The listing builds one solid part. Answer for the finished solid, in the listing's coordinates (mm). A direction names the side the tool comes from. Coordinates: 2 decimals unless noted, no trailing zeros. Loops run counter-clockwise (first coordinate to the right, second up) from the corner with the lowest first, then second, coordinate; pieces in that order, holes last. Notation, with made-up numbers: M 38.5,23 L 97.5,23 A12 ccw 97.5,29 Z; hole C 25,69 d4. An arc over 180 degrees is marked long. Answer as a JSON object with one key per item and string values. Group by question number.
1. A cutting plane is placed at A-A on z = 15.5. Give the vertices of the cut face in (x, y), and give its area (3 significant figures).
2. A cutting plane is placed at C-C on x = -2.1. Give the vertices of the cut face in (y, z).
3. A cutting plane is placed at D-D on y = 2.5. Give the vertices of the cut face in (x, z).
4. Straight lines are drawn through the part: L1, parallel to Z at x = -0.6, y = 1.5; L2, parallel to Y at x = 0.7, z = 6.75; L3, parallel to Z at x = 0.1, y = 0.25. For each, find the intervals that lie inside material, in ascending order.
5. A cutting plane is placed at B-B on y = 0. Give the vertices of the cut face in (x, z), and give its area (3 significant figures).
6. Determine the mould class of faces 1 (the face through (0, 2, 6)), 2 (the face through (-1.5, 0.07, 3.08)), 3 (the face through (-0.27, -1.22, 13.4)), 4 (the face through (1.405, -2.48, 13.395)) for opening direction Y: released by +Y, released by -Y, zero draft, split by the parting line, or undercut.
7. For faces 5 (the face through (2.85, 0, 13)), 6 (the face through (0, 0, 6)), determine the directions among +Z, -Z, +X, -X, +Y, -Y from which every point of the face is accessible in a straight line to the end or side of a thin tool.
from build123d import *

# Parameters (mm, degrees)
SKETCH_R     = 1.5
PAD_DEPTH    = 6
SKETCH001_R  = 1.25
PAD001_DEPTH = 15
CHAMFER_SIZE = 0.25


with BuildPart() as part:
    # Sketch → Pad (new body)
    with BuildSketch(Plane.XY):
        Circle(SKETCH_R)
    extrude(amount=PAD_DEPTH)

    # Sketch001 (on Face3 of Pad) → Pad001 (join)
    with BuildSketch(Plane.XY.offset(6)):
        Polygon((0, -3.290897), (2.85, -1.645448), (2.85, 1.645448), (0, 3.290897), (-2.85, 1.645448), (-2.85, -1.645448), align=None)
        Circle(SKETCH001_R, mode=Mode.SUBTRACT)
    extrude(amount=PAD001_DEPTH)

    # Chamfer
    chamfer_edges = [part.edges().sort_by_distance(p)[0] for p in [
        (-1.5, 0, 0),
    ]]
    chamfer(chamfer_edges, length=CHAMFER_SIZE)


solid = part.part
From the geometry:
{
 "1": {"outline": "M -2.85,-1.65 L 0,-3.29 L 2.85,-1.65 L 2.85,1.65 L 0,3.29 L -2.85,1.65 Z; hole C 0,0 d2.5", "area": "23.2 mm²"},
 "2": {"outline": "M -2.08,6 L 2.08,6 L 2.08,21 L -2.08,21 Z"},
 "3": {"outline": "M -1.37,6 L 1.37,6 L 1.37,21 L -1.37,21 Z"},
 "4": {"L1": "z = 6 to 21", "L2": "y = -2.89 to -1.04, 1.04 to 2.89", "L3": "z = 0 to 6"},
 "5": {"outline": "M -2.85,6 L -1.5,6 L -1.5,0.25 L -1.25,0 L 1.25,0 L 1.5,0.25 L 1.5,6 L 2.85,6 L 2.85,21 L 1.25,21 L 1.25,6 L -1.25,6 L -1.25,21 L -2.85,21 Z", "area": "65.9 mm²"},
 "6": {"face 1": "zero draft", "face 2": "split by the parting line", "face 3": "undercut", "face 4": "released by -Y"},
 "7": {"face 5": "+Z, -Z, +X, +Y, -Y", "face 6": "+Z"}
}
